Check sheet for the modelled part. Datum: model origin and axes. Units: mm. A direction names the side the tool comes from. Give positions to 0.01 mm unless a question says otherwise; leave off trailing zeros. Order: outer loops, then holes, each group sorted by start corner. A loop starts at its lowest first (then second) coordinate and runs counter-clockwise, first axis right, second up. Notation, with made-up numbers: (-24.5, -28.5) -> (-15.5, -28.5) arc R28 cw to (-15.5, 2.5) -> close; hole circle Ø8 at (14.5, 13). An arc over 180 degrees is marked (long way). Answer in a Markdown table with one row per item. Add a question column.
(1) Release check for a two-part mould opening along X. For faces 3 (the face through (11.1, -20.5, 3)), 4 (the face through (0, 0, 3)), 5 (the face through (-2.994, 22.804, 6.295)) record: released by +X, released by -X, zero draft, split by the parting line, or undercut.
(2) Go/stop test with flat-tipped pins: pin 1 (12 mm diameter, centred on x = 2.5, y = 2, fed in from +Z); pin 2 (3 mm diameter, centred on y = 3, z = 7.5, fed in from -X); pin 3 (25 mm diameter, centred on x = -2, y = 4.5, fed in from +Z). Record where each tip stops, or that it passes through.
(3) Set-up check for faces 1 (the face through (-2.799, 21.317, 10.013)), 2 (the face through (-5.47, -24.65, 2.77)): record each of +Z, -Z, +X, -X, +Y, -Y from which the full face is reachable in a straight line by a thin tool's end or side.
(4) Cross-section at D-D (z = 1.5). Record the cut outline in (x, y), then the cut area to 3 significant figures.
(5) Cross-section at B-B (x = 0). Record the cut outline in (y, z).
(6) Thickness scan on L1, parallel to Z at x = -8, y = 8; L2, parallel to Y at x = 0, z = 10.6; L3, parallel to Y at x = 0, z = 10.3. Record the ranges inside material, lowest first. Write a range as [from, to].
(7) Cross-section at A-A (z = 9). Record the cut outline in (x, y).
```python
from build123d import *

# Parameters (mm, degrees)
F0_R     = 25.25
F1_DEPTH = 3
F2_R     = 23
F2_R_2   = 21.5
F3_DEPTH = 9
F4_R     = 2.54
F6_R     = 5.08


# Not quite as in the source:
# - a fillet or chamfer that OpenCascade refuses, or shapes differently, is made with other operations: its cross-section is extruded or revolved along the edge and cut away or added


with BuildPart() as f1:
    # F0 (on Top) → F1 (new body)
    with BuildSketch(Plane.XY):
        Circle(F0_R)
    extrude(amount=F1_DEPTH)

    # F2 (on face) → F3 (join)
    with BuildSketch(Plane.XY.offset(3)):
        Circle(F2_R)
        Circle(F2_R_2, mode=Mode.SUBTRACT)
    extrude(amount=F3_DEPTH)

    # F4
    f4_edges = [f1.edges().sort_by_distance(p)[0] for p in [
        (-25.25, 0, 0),
    ]]
    fillet(f4_edges, radius=F4_R)

    # F5: fillet of radius 2.54 on 1 edges, made by hand

    # F5_s1 → F5_t2 (revolve, cut)
    with BuildSketch(Plane.XZ):
        with BuildLine():
            ThreePointArc((23, 9.6826739547), (22.5922757795, 11.0628913289), (21.5, 12))
            Line((21.5, 12), (23, 12))
            Line((23, 12), (23, 9.6826739547))
        make_face()
    revolve(axis=Axis((0, 0, 12), (0, 0, 1)), mode=Mode.SUBTRACT)

    # F6
    f6_edges = [f1.edges().sort_by_distance(p)[0] for p in [
        (-21.5, 0, 3),
    ]]
    fillet(f6_edges, radius=F6_R)


solid = f1.part
```
Answer below:
| question | item | result |
|---|---|---|
| 1 | face 3 | zero draft |
| 1 | face 4 | undercut |
| 1 | face 5 | split by the parting line |
| 2 | pin 1 | stops at z = 3 |
| 2 | pin 2 | stops at x = -22.95 |
| 2 | pin 3 | stops at z = 3.1 |
| 3 | face 1 | +Z |
| 3 | face 2 | +Z, -Z |
| 4 | outline | circle Ø50.05 at (0, 0) |
| 4 | area | 1,970 mm² |
| 5 | outline | (-25.25, 2.54) arc R2.54 ccw to (-22.71, 0) -> (22.71, 0) arc R2.54 ccw to (25.25, 2.54) -> (25.25, 3) -> (23, 3) -> (23, 9.68) arc R2.54 ccw to (21.5, 12) -> (21.5, 8.08) arc R5.08 cw to (16.42, 3) -> (-16.42, 3) arc R5.08 cw to (-21.5, 8.08) -> (-21.5, 12) arc R2.54 ccw to (-23, 9.68) -> (-23, 3) -> (-25.25, 3) -> close |
| 6 | L1 | z = [0, 3] |
| 6 | L2 | y = [-22.83, -21.5], [21.5, 22.83] |
| 6 | L3 | y = [-22.92, -21.5], [21.5, 22.92] |
| 7 | outline | circle Ø46 at (0, 0); hole circle Ø43 at (0, 0) |
